```python
from build123d import *

# Parameters (mm, degrees)
SKETCH048_W     = 47
SKETCH048_H     = 47
PAD020_DEPTH    = 18.8
SKETCH049_R     = 4
POCKET020_DEPTH = 18.801
SKETCH077_R     = 12
POCKET032_DEPTH = 9


with BuildPart() as part:
    # Sketch048 (on Face8 of ShapeBinder008) → Pad020 (new body)
    with BuildSketch(Plane(origin=(0, 0, -24), x_dir=(-1, 0, 0), z_dir=(0, 0, -1))):
        Rectangle(SKETCH048_W, SKETCH048_H)
    extrude(amount=PAD020_DEPTH)

    # Sketch049 (on Face6 of Pad020) → Pocket020 (cut, through all)
    with BuildSketch(Plane(origin=(0, 0, -42.8), x_dir=(-1, 0, 0), z_dir=(0, 0, -1))):
        Circle(SKETCH049_R)
    extrude(amount=-POCKET020_DEPTH, mode=Mode.SUBTRACT)

    # Sketch077 (on Face5 of Pocket020) → Pocket032 (cut)
    with BuildSketch(Plane(origin=(0, 0, -42.8), x_dir=(-1, 0, 0), z_dir=(0, 0, -1))):
        Circle(SKETCH077_R)
    extrude(amount=-POCKET032_DEPTH, mode=Mode.SUBTRACT)


solid = part.part
```
Input: part model. Units: mm. Frame: model coordinates. A direction names the side the tool comes from. Coordinates: 2 decimals unless noted, no trailing zeros. Write each loop counter-clockwise with the first axis right and the second up, starting at its lowest first coordinate (ties: lowest second). Pieces come first, ordered by that corner, then holes.
1) Section B-B on z = -37.5. Output: boundary loops of the cut face in (x, y).
2) Section D-D on x = -11. Output: boundary loops of the cut face in (y, z).
3) Material intervals for line 1 along Y through (x, z) = (0, -29.75); line 2 along Y through (x, z) = (0, -36.75); line 3 along Z through (x, y) = (8, 7), sorted ascending.
4) Section A-A on x = 0. Output: boundary loops of the cut face in (y, z).
5) Mould query, pull axis X, two halves, no side actions, for faces 1 (the cylindrical face through (0.867, -3.905, -28.969)), 2 (the flat face through (-23.5, 0, -33)), 3 (the flat face through (11, 6, -42.8)). Classes: pulls with the +X half, pulls with the -X half, needs draft (parallel to the pull), parting line crosses it, or undercut.
6) Pin query (flat end, axial travel): pin 1 Ø7 at (x, y) = (4.5, -3) entering from -Z. Return the tip coordinate at first contact, or that it passes through.
7) Set-up query: faces 4 (the flat face through (0, -23.5, -33)), 5 (the flat face through (3, 3, -33.8)). Return all of +Z, -Z, +X, -X, +Y, -Y with unobstructed straight access to the full face (end or side cutting, diameter ignored); none if empty.
Check result:
1. outline: (-23.5, -23.5) - (23.5, -23.5) - (23.5, 23.5) - (-23.5, 23.5) - close; hole circle Ø24 at (0, 0)
2. outline: (-23.5, -42.8) - (-4.8, -42.8) - (-4.8, -33.8) - (4.8, -33.8) - (4.8, -42.8) - (23.5, -42.8) - (23.5, -24) - (-23.5, -24) - close
3. line 1: y = -23.5 to -4, 4 to 23.5
3. line 2: y = -23.5 to -12, 12 to 23.5
3. line 3: z = -33.8 to -24
4. outline: (-23.5, -42.8) - (-12, -42.8) - (-12, -33.8) - (-4, -33.8) - (-4, -24) - (-23.5, -24) - close; (4, -33.8) - (12, -33.8) - (12, -42.8) - (23.5, -42.8) - (23.5, -24) - (4, -24) - close
5. face 1: undercut
5. face 2: pulls with the -X half
5. face 3: needs draft
6. pin 1: stops at z = -33.8
7. face 4: +Z, -Z, +X, -X, -Y
7. face 5: -Z
